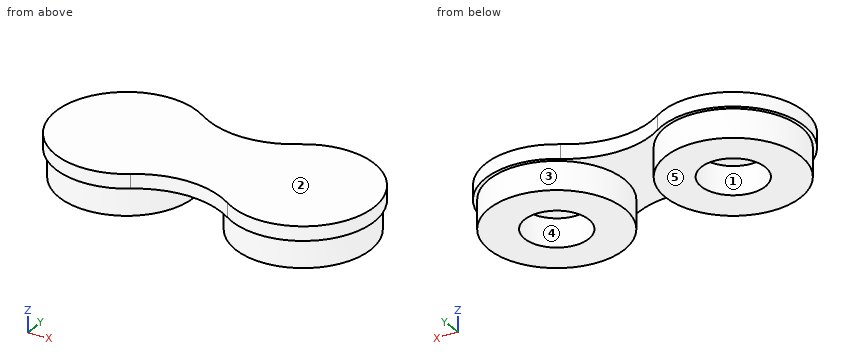
```python
from build123d import *

# Parameters (mm, degrees)
SKETCH1_R             = 4.75
BOSS_EXTRUDE1_DEPTH   = 2
BOSS_EXTRUDE1_2_DEPTH = 2
SKETCH2_R             = 2.25
CUT_EXTRUDE1_DEPTH    = 2
SKETCH2_4_R           = 2.25
CUT_EXTRUDE2_DEPTH    = 2
BOSS_EXTRUDE2_DEPTH   = 1


with BuildPart() as part:
    # Sketch1 → Boss-Extrude1 (new body)
    with BuildSketch(Plane.XY):
        with Locations((-6.15, 0)):
            Circle(SKETCH1_R)
    extrude(amount=BOSS_EXTRUDE1_DEPTH)

    # Sketch2 → Cut-Extrude1 (cut)
    with BuildSketch(Plane.XY.offset(2)):
        with Locations((-6.15, 0)):
            Circle(SKETCH2_R)
    extrude(amount=-CUT_EXTRUDE1_DEPTH, mode=Mode.SUBTRACT)



with BuildPart() as body_2:
    # Sketch1 → Boss-Extrude1 2 (new body)
    with BuildSketch(Plane.XY):
        with Locations(Location((6.15, 0, 0), (0, 0, 180))):
            Circle(SKETCH1_R)
    extrude(amount=BOSS_EXTRUDE1_2_DEPTH)

    # Sketch2_4 → Cut-Extrude2 (cut)
    with BuildSketch(Plane.XY.offset(2)):
        with Locations((6.15, 0)):
            Circle(SKETCH2_4_R)
    extrude(amount=-CUT_EXTRUDE2_DEPTH, mode=Mode.SUBTRACT)


with BuildPart() as part_1:
    add(part.part)

    add(body_2.part)  # Boss-Extrude2 merges body 2
    # Sketch4 → Boss-Extrude2 (add)
    with BuildSketch(Plane.XY.offset(2)):
        with BuildLine():
            ThreePointArc((-3.367629676, 4.1543249), (-11.15, 3.6455e-05), (-3.367690254, -4.154365473))
            ThreePointArc((-3.367690254, -4.154365473), (0, -3.130814748), (3.367690254, -4.154365473))
            ThreePointArc((3.367690254, -4.154365473), (11.15, 3.6455e-05), (3.367629676, 4.1543249))
            ThreePointArc((3.367629676, 4.1543249), (0, 3.130765766), (-3.367629676, 4.1543249))
        make_face()
    extrude(amount=BOSS_EXTRUDE2_DEPTH)


solid = part_1.part
```
Can you work these out from the model? Positions are in its coordinate system, mm. Face numbers are marked on the shaded views. A direction names the side the tool comes from. Give positions to 0.01 mm unless a question says otherwise; leave off trailing zeros. Write each loop counter-clockwise with the first axis right and the second up, starting at its lowest first coordinate (ties: lowest second). Pieces come first, ordered by that corner, then holes. Notation, with made-up numbers: (18, -15) -> (26, -15) arc R11 ccw to (26, 5) -> close; hole circle Ø1 at (44.5, 85.5). An arc over 180 degrees is marked (long way). Write item = value, one per line.
(1) For the marked faces 1 and 2, which set-ups out of +Z, -Z, +X, -X, +Y, -Y let a thin tool reach every point of the face, with its end or its side?
Worked out:
face_1 = -Z
face_2 = +Z, +X, -X, +Y, -Y
(2) I need wall thicknesses on probe 1 along Y at (x, z) = (6.15, 0.8); probe 2 along X at (y, z) = (1.75, 1.3); probe 3 along X at (y, z) = (-2, 1.95). Which ranges of each line are inside material? Lowest first, please. Write a range as from..to.
Worked out:
probe_1 = -4.75..-2.25, 2.25..4.75
probe_2 = -10.57..-7.56, -4.74..-1.73, 1.73..4.74, 7.56..10.57
probe_3 = -10.46..-7.18, -5.12..-1.84, 1.84..5.12, 7.18..10.46
(3) Suppose I cut it at C-C on x = -6.15. Write out the boundary of the cut face in (y, z).
Worked out:
outline = (-5, 2) -> (-4.75, 2) -> (-4.75, 0) -> (-2.25, 0) -> (-2.25, 2) -> (2.25, 2) -> (2.25, 0) -> (4.75, 0) -> (4.75, 2) -> (5, 2) -> (5, 3) -> (-5, 3) -> close
(4) Suppose I cut it at D-D on x = 2.75. Write out the boundary of the cut face in (y, z), then the cut area to 3 significant figures.
Worked out:
outline = (-3.79, 2) -> (-3.32, 2) -> (-3.32, 0) -> (3.32, 0) -> (3.32, 2) -> (3.79, 2) -> (3.79, 3) -> (-3.79, 3) -> close
area = 20.9 mm^2
(5) Suppose I cut it at A-A on y = 0. Write out the boundary of the cut face in (x, z), then the cut area to 3 significant figures.
Worked out:
outline = (-11.15, 2) -> (-10.9, 2) -> (-10.9, 0) -> (-8.4, 0) -> (-8.4, 2) -> (-3.9, 2) -> (-3.9, 0) -> (-1.4, 0) -> (-1.4, 2) -> (1.4, 2) -> (1.4, 0) -> (3.9, 0) -> (3.9, 2) -> (8.4, 2) -> (8.4, 0) -> (10.9, 0) -> (10.9, 2) -> (11.15, 2) -> (11.15, 3) -> (-11.15, 3) -> close
area = 42.3 mm^2
(6) Thinking about a two-plate mould opening in X: for the marked faces 3, 4 and 5, which applies, released by +X, released by -X, zero draft, split by the parting line, or undercut?
Worked out:
face_3 = undercut
face_4 = undercut
face_5 = zero draft
(7) I'm going to push flat-ended pins straight in: P1, Ø1, axis at x = 5.5, z = 0.5, coming from the +Y side; P2, Ø1, axis at x = -8.5, y = 2, coming from the -Z side; P3, Ø1.5, axis at x = 7.5, z = 2.5, coming from the +Y side; P4, Ø1.5, axis at y = -1.5, z = 2, coming from the -X side. Where does each tip first touch, or does it pass through?
Worked out:
P1 = 4.75
P2 = 0
P3 = 4.96
P4 = -11.09
(8) Suppose I cut it at B-B on z = 1.1. Write out the boundary of the cut face in (x, y), then the cut area to 3 significant figures.
Worked out:
outline = circle Ø9.5 at (-6.15, 0); circle Ø9.5 at (6.15, 0); hole circle Ø4.5 at (-6.15, 0); hole circle Ø4.5 at (6.15, 0)
area = 110 mm^2
